Work out the finished part from the listing and answer in its coordinate system (mm). A direction names the side the tool comes from. Round coordinates to 2 decimals unless told otherwise and drop trailing zeros. Order: outer loops, then holes, each group sorted by start corner. A loop starts at its lowest first (then second) coordinate and runs counter-clockwise, first axis right, second up. Notation, with made-up numbers: (24.25, -31.5) -> (77.25, -31.5) arc R20 ccw to (77.25, -24.5) -> close; hole circle Ø8 at (80, -8). An arc over 180 degrees is marked (long way). Use a Markdown table: item, result. Add a question column.
Item 1: A cutting plane is placed at A-A, the plane z = 17.5. Determine the outline of the cut face in (x, y), plus the area to 3 significant figures.
Item 2: A cutting plane is placed at D-D, the plane x = -48.5. Determine the outline of the cut face in (y, z), plus the area to 3 significant figures.
Item 3: Find the intervals of material crossed by L1, parallel to X at y = 1, z = 13.5; L2, parallel to Z at x = -85, y = -11.75; L3, parallel to X at y = 3.25, z = -35, in increasing order. Write a range as [from, to].
Item 4: A cutting plane is placed at B-B, the plane x = -92.5. Determine the outline of the cut face in (y, z), plus the area to 3 significant figures.
Item 5: A cutting plane is placed at C-C, the plane y = 0. Determine the outline of the cut face in (x, z), plus the area to 3 significant figures.
Item 6: Flat-ended cylindrical pins translate along their axes: P1, Ø8, axis at y = -10, z = 79, coming from the -X side; P2, Ø3, axis at y = -0.5, z = 58.5, coming from the +X side; P3, Ø3, axis at x = -40.5, y = 1, coming from the +Z side. Find the tip coordinate at first contact, or state that the pin passes through.
Item 7: A tool of negligible diameter and unlimited length cuts with its end or side. For faces 4 (the flat face through (-91, 0, -22.175)), 5 (the flat face through (-30, 3, 22)), 6 (the flat face through (-20.113, 0, 15)), from which of +Z, -Z, +X, -X, +Y, -Y can it reach the whole face along a straight path? Write none if from no direction.
Item 8: For a pull along Z with two mould halves and no side action, classify faces 1 (the cylindrical face through (-18.419, 0.042, 3.744)), 2 (the flat face through (-40, 0, 30.458)), 3 (the cylindrical face through (-105.214, 0.21, 118.157)) as +Z half, -Z half, draft (parallel to the pull), parting line (faces both ways), or undercut.
from build123d import *

# Parameters (mm, degrees)
BOSS_EXTRUDE1_DEPTH      = 15
BOSS_EXTRUDE1_DEPTH_BACK = 15
BOSS_EXTRUDE2_DEPTH      = 3
BOSS_EXTRUDE2_DEPTH_BACK = 3
FILLET1_R                = 10
FILLET2_R                = 5


with BuildPart() as part:
    # Sketch1 → Boss-Extrude1 (new, two sides: drawn at the far end of the back side and taken through both)
    with BuildSketch(Plane(origin=(0, 0, 0), x_dir=(1, 0, 0), z_dir=(0, 1, 0)).offset(-BOSS_EXTRUDE1_DEPTH_BACK)):
        Polygon((-106.717200023, 22.174603175), (-106.717200023, 45.125781111), (-55.917200023, 45.125781111), (-55.917200023, -139.682824762), (-106.717200023, -139.682824762), (-106.717200023, -116.731646825), (-81.317200023, -116.731646825), (-81.317200023, 22.174603175), align=None)
    extrude(amount=BOSS_EXTRUDE1_DEPTH + BOSS_EXTRUDE1_DEPTH_BACK)

    # Sketch1<3> → Boss-Extrude2 (add, two sides: drawn at the far end of the back side and taken through both)
    with BuildSketch(Plane(origin=(0, 0, 0), x_dir=(1, 0, 0), z_dir=(0, 1, 0)).offset(-BOSS_EXTRUDE2_DEPTH_BACK)):
        Polygon((-55.917200023, -21.59149981), (-55.917200023, -30.457986667), (-13.752700087, -30.457986667), (-13.752700087, 0), (-20.113440658, 0), (-20.113440658, -21.59149981), align=None)
    extrude(amount=BOSS_EXTRUDE2_DEPTH + BOSS_EXTRUDE2_DEPTH_BACK)

    # Fillet1
    # the kernel refuses this fillet: 10 mm, written as the material it takes off along each edge
    with BuildSketch(Plane(origin=(-106.717200023, 40, -45.125781111), x_dir=(0, 0, 1), z_dir=(0, -1, 0)), Plane(origin=(-55.917200023, 40, 139.682824762), x_dir=(0, 0, -1), z_dir=(0, -1, 0)), Plane(origin=(-55.917200023, 40, -45.125781111), x_dir=(-1, 0, 0), z_dir=(0, -1, 0)), Plane(origin=(-106.717200023, 40, 139.682824762), x_dir=(1, 0, 0), z_dir=(0, -1, 0))) as fillet1_piece_1:
        with BuildLine():
            CenterArc((FILLET1_R, -FILLET1_R), FILLET1_R, 90, 90)
            Line((0, -FILLET1_R), (-FILLET1_R * 0.02, -FILLET1_R))
            Line((-FILLET1_R * 0.02, -FILLET1_R), (-FILLET1_R * 0.02, FILLET1_R * 0.02))
            Line((-FILLET1_R * 0.02, FILLET1_R * 0.02), (FILLET1_R, FILLET1_R * 0.02))
            Line((FILLET1_R, FILLET1_R * 0.02), (FILLET1_R, 0))
        make_face()
    extrude(amount=80, mode=Mode.SUBTRACT)
    with BuildSketch(Plane(origin=(-13.752700087, -28, 30.457986667), x_dir=(-1, 0, 0), z_dir=(0, 1, 0))) as fillet1_piece_2:
        with BuildLine():
            CenterArc((FILLET1_R, -FILLET1_R), FILLET1_R, 90, 90)
            Line((0, -FILLET1_R), (-FILLET1_R * 0.02, -FILLET1_R))
            Line((-FILLET1_R * 0.02, -FILLET1_R), (-FILLET1_R * 0.02, FILLET1_R * 0.02))
            Line((-FILLET1_R * 0.02, FILLET1_R * 0.02), (FILLET1_R, FILLET1_R * 0.02))
            Line((FILLET1_R, FILLET1_R * 0.02), (FILLET1_R, 0))
        make_face()
    extrude(amount=56, mode=Mode.SUBTRACT)
    with BuildSketch(Plane(origin=(-20.113440658, 26.285697167, 0), x_dir=(1, 0, 0), z_dir=(0, -1, 0))) as fillet1_piece_3:
        with BuildLine():
            CenterArc((10, 9.314278867), FILLET1_R, 180, 68.658501665)
            Line((0, 9.314278867), (-0.2, 9.314278867))
            Line((-0.2, 9.314278867), (-0.2, 0))
            Line((-0.2, 0), (0, -0.2))
            ThreePointArc((0, -0.2), (3.180370286, -0.2), (6.287955383, -0.186285577))
            Line((6.287955383, -0.186285577), (6.360740571, 0))
        make_face()
    extrude(amount=52.571394335, mode=Mode.SUBTRACT)

    # Fillet2
    fillet2_edges = [part.edges().sort_by_distance(p)[0] for p in [
        (-106.717200023, 0, 116.731646825),
        (-106.717200023, 0, -22.174603175),
    ]]
    fillet(fillet2_edges, radius=FILLET2_R)


solid = part.part
Reported:
| question | item | result |
|---|---|---|
| 1 | outline | (-81.32, -15) -> (-55.92, -15) -> (-55.92, 15) -> (-81.32, 15) -> close; (-20.11, -3) -> (-13.75, -3) -> (-13.75, 3) -> (-20.11, 3) -> close |
| 1 | area | 800 mm² |
| 2 | outline | (-3, 21.59) -> (3, 21.59) -> (3, 30.46) -> (-3, 30.46) -> close |
| 2 | area | 53.2 mm² |
| 3 | L1 | [-81.32, -55.92], [-20.11, -13.75] |
| 3 | L2 | [-45.13, -22.17], [116.73, 139.68] |
| 3 | L3 | [-106.72, -55.92] |
| 4 | outline | (-15, -45.13) -> (15, -45.13) -> (15, -22.17) -> (-15, -22.17) -> close; (-15, 116.73) -> (15, 116.73) -> (15, 139.68) -> (-15, 139.68) -> close |
| 4 | area | 1,380 mm² |
| 5 | outline | (-106.72, -35.13) arc R10 ccw to (-96.72, -45.13) -> (-65.92, -45.13) arc R10 ccw to (-55.92, -35.13) -> (-55.92, 21.59) -> (-20.11, 21.59) -> (-20.11, 9.31) arc R10 ccw to (-13.75, 0) -> (-13.75, 20.46) arc R10 ccw to (-23.75, 30.46) -> (-55.92, 30.46) -> (-55.92, 129.68) arc R10 ccw to (-65.92, 139.68) -> (-96.72, 139.68) arc R10 ccw to (-106.72, 129.68) -> (-106.72, 121.73) arc R5 ccw to (-101.72, 116.73) -> (-81.32, 116.73) -> (-81.32, -22.17) -> (-101.72, -22.17) arc R5 ccw to (-106.72, -27.17) -> close |
| 5 | area | 6,240 mm² |
| 6 | P1 | x = -81.32 |
| 6 | P2 | x = -55.92 |
| 6 | P3 | z = 30.46 |
| 7 | face 4 | -X, +Y, -Y |
| 7 | face 5 | +Z, -Z, +X, +Y |
| 7 | face 6 | -Z, +Y, -Y |
| 8 | face 1 | -Z half |
| 8 | face 2 | +Z half |
| 8 | face 3 | undercut |
